```python
from build123d import *

# Parameters (mm, degrees)
SKETCH8_W            = 54
SKETCH8_H            = 25
BOSS_EXTRUDE1_DEPTH  = 11
SKETCH9_W            = 20
SKETCH9_H            = 21.5
CUT_EXTRUDE1_DEPTH   = 10
SKETCH11_W           = 8
SKETCH11_H           = 8
CUT_EXTRUDE5_DEPTH   = 3.5
JOYSTICK_ENTRY_REACH = 40.406
SKETCH10_W           = 16.4
SKETCH10_H           = 8.2
SKETCH13_W           = 16
SKETCH13_H           = 2.5
CUT_EXTRUDE6_DEPTH   = 8


with BuildPart() as part:
    # Sketch8 → Boss-Extrude1 (new body)
    with BuildSketch(Plane(origin=(0, 0, 0), x_dir=(1, 0, 0), z_dir=(0, 1, 0))):
        with Locations((0, 13)):
            Rectangle(SKETCH8_W, SKETCH8_H)
    extrude(amount=BOSS_EXTRUDE1_DEPTH)

    # Sketch9 → Cut-Extrude1 (cut)
    with BuildSketch(Plane(origin=(0, 11, 0), x_dir=(1, 0, 0), z_dir=(0, 1, 0))):
        with Locations((-15, 12.75)):
            Rectangle(SKETCH9_W, SKETCH9_H)
    extrude(amount=-CUT_EXTRUDE1_DEPTH, mode=Mode.SUBTRACT)

    # Sketch11 → Cut-Extrude5 (cut)
    with BuildSketch(Plane(origin=(0, 11, 0), x_dir=(1, 0, 0), z_dir=(0, 1, 0))):
        with Locations((18, 4.5)):
            Rectangle(SKETCH11_W, SKETCH11_H)
    extrude(amount=-CUT_EXTRUDE5_DEPTH, mode=Mode.SUBTRACT)

    # Sketch10 → Joystick Entry (cut, up to next)
    with BuildSketch(Plane.XY.offset(-0.5), mode=Mode.PRIVATE) as joystick_entry_sk1:
        with Locations((-15, 5.1)):
            Rectangle(SKETCH10_W, SKETCH10_H)
    joystick_entry_tool1 = extrude(joystick_entry_sk1.sketch, amount=-JOYSTICK_ENTRY_REACH, mode=Mode.PRIVATE) & part.part
    add(joystick_entry_tool1.solids().sort_by_distance((-15, 5.1, -0.5))[0], mode=Mode.SUBTRACT)

    # Sketch13 → Cut-Extrude6 (cut)
    with BuildSketch(Plane.XY.offset(-0.5)):
        with Locations((17.5, 8.75)):
            Rectangle(SKETCH13_W, SKETCH13_H)
    extrude(amount=-CUT_EXTRUDE6_DEPTH, mode=Mode.SUBTRACT)


solid = part.part
```
Part model, mm, in its own coordinate system. A direction names the side the tool comes from. Coordinates: 2 decimals unless noted, no trailing zeros. Order: outer loops, then holes, each group sorted by start corner. A loop starts at its lowest first (then second) coordinate and runs counter-clockwise, first axis right, second up. Notation, with made-up numbers: (8.25, 20) - (25.25, 20) arc R27 cw to (25.25, 54) - close; hole circle Ø9 at (-2.75, 23). An arc over 180 degrees is marked (long way). Return JSON: item names as keys, results as strings. Group by question number.
Item 1: Cut at B-B (x = 13.5). List the corners of the cut face in (y, z).
Item 2: Cut at C-C (z = -6). List the corners of the cut face in (x, y), plus the area to 3 significant figures.
Item 3: Which spindle directions (+Z, -Z, +X, -X, +Y, -Y) get a long thin tool onto all of the face, cutting with end or side? Do faces 1 (the face through (14, 10.5, -4.4)), 2 (the face through (25.5, 9, -4)), 3 (the face through (-15.1, 9.4, -2)). Say none if no direction does.
Item 4: Pin check, flat tips, straight feed: pin 1 (6.5 mm diameter, centred on x = 17, z = -5.5, fed in from +Y); pin 2 (1.8 mm diameter, centred on x = 18, y = 9, fed in from +Z). Stop position of each tip, or through.
Item 5: Drill centre lines: probe 1 along X at (y, z) = (8.25, -5.5); probe 2 along X at (y, z) = (7.5, -13); probe 3 along Y at (x, z) = (13, -3). Where is each one in solid material? Low to high. Write a range as from..to.
Item 6: Pull direction X, two halves, no side cores. Call faces 4 (the face through (-25, 6, -13)), 5 (the face through (27, 5, -13)), 6 (the face through (0, 5, -0.5)): pulls with the +X half, pulls with the -X half, needs draft (parallel to the pull), parting line crosses it, or undercut.
Item 7: Cut at D-D (y = 8.5). List the corners of the cut face in (x, z), plus the area to 3 significant figures.
Item 8: Cut at A-A (x = -15). List the corners of the cut face in (y, z), plus the area to 3 significant figures.
Check values:
{
 "1": {"outline": "(0, -25.5) - (11, -25.5) - (11, -0.5) - (10, -0.5) - (10, -8.5) - (7.5, -8.5) - (7.5, -0.5) - (0, -0.5) - close"},
 "2": {"outline": "(-27, 0) - (27, 0) - (27, 11) - (22, 11) - (22, 10) - (25.5, 10) - (25.5, 7.5) - (9.5, 7.5) - (9.5, 10) - (14, 10) - (14, 11) - (-5, 11) - (-5, 1) - (-25, 1) - (-25, 11) - (-27, 11) - close", "area": "346 mm2"},
 "3": {"face 1": "+Z, +Y", "face 2": "+Z", "face 3": "+Y"},
 "4": {"pin 1": "stops at y = 11", "pin 2": "stops at z = -8.5"},
 "5": {"probe 1": "x = -27..-25, -5..9.5, 25.5..27", "probe 2": "x = -27..-25, -5..27", "probe 3": "y = 0..7.5, 10..11"},
 "6": {"face 4": "undercut", "face 5": "pulls with the +X half", "face 6": "needs draft"},
 "7": {"outline": "(-27, -25.5) - (27, -25.5) - (27, -0.5) - (25.5, -0.5) - (25.5, -8.5) - (9.5, -8.5) - (9.5, -0.5) - (-6.8, -0.5) - (-6.8, -2) - (-5, -2) - (-5, -23.5) - (-25, -23.5) - (-25, -2) - (-23.2, -2) - (-23.2, -0.5) - (-27, -0.5) - close", "area": "767 mm2"},
 "8": {"outline": "(0, -25.5) - (11, -25.5) - (11, -23.5) - (1, -23.5) - (1, -0.5) - (0, -0.5) - close; (9.2, -2) - (11, -2) - (11, -0.5) - (9.2, -0.5) - close", "area": "47.7 mm2"}
}
